```python
from build123d import *

# Parameters (mm, degrees)
EXTRUDE_1_DEPTH     = 17
EXTRUDE_2_DEPTH     = 1
SKETCH_3_W          = 13.083033948
SKETCH_3_H          = 19
CUT_EXTRUDE_1_DEPTH = 16
SKETCH_4_W          = 26.5
SKETCH_4_H          = 3
CUT_EXTRUDE_2_DEPTH = 26
SKETCH_5_W          = 9.5
SKETCH_5_H          = 3
CUT_EXTRUDE_3_DEPTH = 26
FILLET_1_R          = 2


with BuildPart() as part:
    # Эскиз1 → Бобышка-Вытянуть1 (new body)
    with BuildSketch(Plane(origin=(0, 0, 0), x_dir=(1, 0, 0), z_dir=(0, 1, 0))):
        with BuildLine():
            Line((38.5, 10.5), (-43.5, 10.5))
            Line((-43.5, 10.5), (-43.5, -10.5))
            Line((-43.5, -10.5), (38.5, -10.5))
            ThreePointArc((38.5, -10.5), (42.035533906, -9.035533906), (43.5, -5.5))
            Line((43.5, -5.5), (43.5, 5.5))
            ThreePointArc((43.5, 5.5), (42.035533906, 9.035533906), (38.5, 10.5))
        make_face()
        with BuildLine():
            Line((-42.5, 9.5), (-42.5, -9.5))
            Line((-42.5, -9.5), (38.5, -9.5))
            ThreePointArc((38.5, -9.5), (41.328427125, -8.328427125), (42.5, -5.5))
            Line((42.5, -5.5), (42.5, 5.5))
            ThreePointArc((42.5, 5.5), (41.328427125, 8.328427125), (38.5, 9.5))
            Line((38.5, 9.5), (-42.5, 9.5))
        make_face(mode=Mode.SUBTRACT)
    extrude(amount=EXTRUDE_1_DEPTH)

    # Эскиз2 → Бобышка-Вытянуть2 (add)
    with BuildSketch(Plane.XZ):
        with BuildLine():
            Line((-43.5, 10.5), (-43.5, -10.5))
            Line((-43.5, -10.5), (38.5, -10.5))
            ThreePointArc((38.5, -10.5), (42.035533906, -9.035533906), (43.5, -5.5))
            Line((43.5, -5.5), (43.5, 5.5))
            ThreePointArc((43.5, 5.5), (42.035533906, 9.035533906), (38.5, 10.5))
            Line((38.5, 10.5), (-43.5, 10.5))
        make_face()
    extrude(amount=-EXTRUDE_2_DEPTH)

    # Эскиз3 → Вырез-Вытянуть1 (cut)
    with BuildSketch(Plane(origin=(0, 17, 0), x_dir=(1, 0, 0), z_dir=(0, 1, 0))):
        with Locations((-45.110446102, 0)):
            Rectangle(SKETCH_3_W, SKETCH_3_H)
    extrude(amount=-CUT_EXTRUDE_1_DEPTH, mode=Mode.SUBTRACT)

    # Эскиз4 → Вырез-Вытянуть2 (cut)
    with BuildSketch(Plane.XY.offset(10.5)):
        with Locations((30.25, 15.5)):
            Rectangle(SKETCH_4_W, SKETCH_4_H)
    extrude(amount=-CUT_EXTRUDE_2_DEPTH, mode=Mode.SUBTRACT)

    # Эскиз5 → Вырез-Вытянуть3 (cut)
    with BuildSketch(Plane.XY.offset(10.5)):
        with Locations((-38.75, 15.5)):
            Rectangle(SKETCH_5_W, SKETCH_5_H)
    extrude(amount=-CUT_EXTRUDE_3_DEPTH, mode=Mode.SUBTRACT)

    # Скругление1
    fillet_1_edges = [part.edges().sort_by_distance(p)[0] for p in [
        (-43.5, 14, -10),
        (-43.5, 14, 10),
    ]]
    fillet(fillet_1_edges, radius=FILLET_1_R)


solid = part.part
```
Can you work these out from the model? Positions are in its coordinate system, mm. A direction names the side the tool comes from. Coordinates: 2 decimals unless noted, no trailing zeros. Order: outer loops, then holes, each group sorted by start corner. A loop starts at its lowest first (then second) coordinate and runs counter-clockwise, first axis right, second up. Notation, with made-up numbers: (46, 24) - (102, 24) arc R29 cw to (102, 49) - close; hole circle Ø10 at (37, 73.25). An arc over 180 degrees is marked (long way). Answer in a Markdown table with one row per item.
1. If we mould it in two halves opening along Z, with no side actions, what happens to faces 1 (the cylindrical face through (41.359, 7.409, -8.297)), 2 (the flat face through (43, 14, 0)), 3 (the flat face through (-3, 8, 10.5)), 4 (the flat face through (-1, 1, 0))? For each: pulls with the +Z half, pulls with the -Z half, needs draft (parallel to the pull), parting line crosses it, or undercut.
Reply:
| item | result |
|---|---|
| face 1 | undercut |
| face 2 | needs draft |
| face 3 | pulls with the +Z half |
| face 4 | undercut |
2. Suppose I cut it at A-A (x = -4). Please give me the cut outline in (y, z).
Reply:
| item | result |
|---|---|
| outline | (0, -10.5) - (17, -10.5) - (17, -9.5) - (1, -9.5) - (1, 9.5) - (17, 9.5) - (17, 10.5) - (0, 10.5) - close |
3. If I drill on line 1 along Z through (x, y) = (-38.5, 3.25); line 2 along Y through (x, z) = (27.5, -0.75); line 3 along X through (y, z) = (4.25, -6.5), over which ranges is the centre line in solid material (lowest first)?
Reply:
| item | result |
|---|---|
| line 1 | z = -10.5 to -9.5, 9.5 to 10.5 |
| line 2 | y = 0 to 1 |
| line 3 | x = 42.37 to 43.4 |
4. Suppose I cut it at B-B (y = 9.5). Please give me the cut outline in (x, z).
Reply:
| item | result |
|---|---|
| outline | (-43.5, -10.5) - (38.5, -10.5) arc R5 ccw to (43.5, -5.5) - (43.5, 5.5) arc R5 ccw to (38.5, 10.5) - (-43.5, 10.5) - (-43.5, 9.5) - (38.5, 9.5) arc R4 cw to (42.5, 5.5) - (42.5, -5.5) arc R4 cw to (38.5, -9.5) - (-43.5, -9.5) - close |
5. Suppose I cut it at C-C (z = -6.25). Please give me the cut outline in (x, y).
Reply:
| item | result |
|---|---|
| outline | (-43.5, 0) - (43.44, 0) - (43.44, 14) - (42.43, 14) - (42.43, 1) - (-43.5, 1) - close |
6. Suppose I cut it at D-D (x = -36). Please give me the cut outline in (y, z).
Reply:
| item | result |
|---|---|
| outline | (0, -10.5) - (14, -10.5) - (14, -9.5) - (1, -9.5) - (1, 9.5) - (14, 9.5) - (14, 10.5) - (0, 10.5) - close |
7. For pin 1 (1 mm diameter, centred on y = 13, z = 1, fed in from -X); pin 2 (0.8 mm diameter, centred on y = 16, z = 10, fed in from -X), each with a flat end and sliding along its axis, tell me the tip position at first contact or that it passes through.
Reply:
| item | result |
|---|---|
| pin 1 | stops at x = 42.5 |
| pin 2 | stops at x = -34 |
8. For faces 5 (the flat face through (-3, 9, 9.5)), 6 (the flat face through (-1, 0, 0)), which set-ups out of +Z, -Z, +X, -X, +Y, -Y let a thin tool reach every point of the face, with its end or its side?
Reply:
| item | result |
|---|---|
| face 5 | -X, +Y |
| face 6 | +Z, -Z, +X, -X, -Y |
